Read the model definition and answer for the solid it produces. Units are mm, in the model's axes. A direction names the side the tool comes from. Coordinates: 2 decimals unless noted, no trailing zeros. Loops run counter-clockwise (first coordinate to the right, second up) from the corner with the lowest first, then second, coordinate; pieces in that order, holes last.
Q1. Section B-B (y = -0.4) is taken. Give the vertices of the cut face in (x, z).
Q2. The mould has two halves that part along X. Classify faces 4 (the face through (12, 0, 2)), 5 (the face through (15, 0, 0.75)): pulls with the +X half, pulls with the -X half, needs draft (parallel to the pull), parting line crosses it, or undercut.
Q3. Straight lines are drawn through the part: line 1 (Z direction, x = 9.5, y = -1.15); line 2 (Z direction, x = -10, y = 0.8); line 3 (X direction, y = -0.7, z = 6.5). For each, find the intervals that lie inside material, in ascending order.
Q4. Which of the six approach directions +Z, -Z, +X, -X, +Y, -Y give full straight-line access (tool end or side, diameter ignored) to faces 1 (the face through (11, 2.33, 1)), 2 (the face through (9.9, -0.03, 1.67)), 3 (the face through (15, 0, -0.75))?
Q5. Flat-ended cylindrical pins translate along their axes: P1, Ø1.5, axis at x = 3.5, y = 1, coming from the +Z side; P2, Ø2, axis at y = 1.5, z = 13, coming from the -X side; P3, Ø2.5, axis at x = 13, y = 1, coming from the +Z side. Find the tip coordinate at first contact, or state that the pin passes through.
Q6. Section A-A (y = 1.8) is taken. Give the vertices of the cut face in (x, z), then the cut area to 3 significant figures.
from build123d import *

# Parameters (mm, degrees)
PAD_DEPTH    = 2.33
SKETCH002_W  = 21.853373
SKETCH002_H  = 1.5
POCKET_DEPTH = 2.5


with BuildPart() as part:
    # Sketch → Revolution (revolve)
    with BuildSketch(Plane.XY):
        with BuildLine():
            ThreePointArc((20.25, -2.331845), (21, 0), (20.25, 2.331845))
            Line((13.75, 2.331845), (20.25, 2.331845))
            ThreePointArc((13.75, 2.331845), (13, 0), (13.75, -2.331845))
            Line((20.25, -2.331845), (13.75, -2.331845))
        make_face()
    revolve(axis=Axis((0, 0, 0), (0, 1, 0)))

    # Sketch001 → Pad (new body, symmetric)
    with BuildSketch(Plane.XZ):
        with BuildLine():
            ThreePointArc((11, 2), (9, 0), (11, -2))
            Line((11, -2), (19, -2))
            ThreePointArc((19, -2), (21, 0), (19, 2))
            Line((19, 2), (11, 2))
        make_face()
    extrude(amount=PAD_DEPTH, both=True)

    # Sketch002 → Pocket (cut, symmetric)
    with BuildSketch(Plane.XZ):
        with Locations((10.926686, 0)):
            Rectangle(SKETCH002_W, SKETCH002_H)
    extrude(amount=POCKET_DEPTH, both=True, mode=Mode.SUBTRACT)


solid = part.part
Numbers:
1. outline: (9.15, -0.75) arc R2 ccw to (11, -2) - (12.87, -2) arc R13.02 cw (long way) to (12.87, 2) - (11, 2) arc R2 ccw to (9.15, 0.75) - (20.97, 0.75) arc R20.98 ccw (long way) to (20.97, -0.75) - close
2. face 4: undercut
2. face 5: needs draft
3. line 1: z = -18.54 to -9.12, -1.32 to -0.75, 0.75 to 1.32, 9.12 to 18.54
3. line 2: z = -18.37 to -8.43, 8.43 to 18.37
3. line 3: x = -19.9 to -11.33, 11.33 to 19.9
4. face 1: +Z, -Z, +X, -X, +Y
4. face 2: +Y, -Y
4. face 3: +X, +Y, -Y
5. P1: stops at z = 20.76
5. P2: stops at x = -16.99
5. P3: stops at z = 17.31
6. outline: (9.15, -0.75) arc R2 ccw to (11, -2) - (13.28, -2) arc R13.43 cw (long way) to (13.28, 2) - (11, 2) arc R2 ccw to (9.15, 0.75) - (20.85, 0.75) arc R2 ccw to (20.53, 1.29) arc R20.57 ccw (long way) to (20.53, -1.29) arc R2 ccw to (20.85, -0.75) - close
6. area: 762 mm2
